Could you check a few things on this model? Use its own coordinates, in mm. Give positions to 0.01 mm unless a question says otherwise; leave off trailing zeros. Order: outer loops, then holes, each group sorted by start corner. A loop starts at its lowest first (then second) coordinate and runs counter-clockwise, first axis right, second up.
from build123d import *

# Parameters (mm, degrees)
EXTRUDE_1_DEPTH = 1.2


with BuildPart() as part:
    # 스케치1 → 보스-돌출1 (new body)
    with BuildSketch(Plane(origin=(0, 0, 0), x_dir=(1, 0, 0), z_dir=(0, 1, 0))):
        with BuildLine():
            Line((96.5, 48.995454452), (96.5, 85))
            ThreePointArc((96.5, 85), (93.863961031, 91.363961031), (87.5, 94))
            Line((87.5, 94), (-96.5, 94))
            Line((-96.5, 94), (-96.5, -95))
            Line((-96.5, -95), (-7.113574645, -95))
            ThreePointArc((-7.113574645, -95), (8.212657599, 3.247727485), (96.5, 48.995454452))
        make_face()
        with BuildLine():
            ThreePointArc((-86, -83), (-88, -81), (-86, -79))
            Line((-86, -79), (-84, -79))
            Line((-84, -79), (-82, -79))
            ThreePointArc((-82, -79), (-80.585786438, -79.585786438), (-80, -81))
            ThreePointArc((-80, -81), (-80.585786438, -82.414213562), (-82, -83))
            Line((-82, -83), (-84, -83))
            Line((-84, -83), (-86, -83))
        make_face(mode=Mode.SUBTRACT)
        with BuildLine():
            ThreePointArc((-86, -61), (-88, -59), (-86, -57))
            Line((-86, -57), (-84, -57))
            Line((-84, -57), (-82, -57))
            ThreePointArc((-82, -57), (-80.585786438, -57.585786438), (-80, -59))
            ThreePointArc((-80, -59), (-80.585786438, -60.414213562), (-82, -61))
            Line((-82, -61), (-84, -61))
            Line((-84, -61), (-86, -61))
        make_face(mode=Mode.SUBTRACT)
        with BuildLine():
            ThreePointArc((-86, 57), (-88, 59), (-86, 61))
            Line((-86, 61), (-84, 61))
            Line((-84, 61), (-82, 61))
            ThreePointArc((-82, 61), (-80.585786438, 60.414213562), (-80, 59))
            ThreePointArc((-80, 59), (-80.585786438, 57.585786438), (-82, 57))
            Line((-82, 57), (-84, 57))
            Line((-84, 57), (-86, 57))
        make_face(mode=Mode.SUBTRACT)
        with BuildLine():
            ThreePointArc((-86, 79), (-88, 81), (-86, 83))
            Line((-86, 83), (-84, 83))
            Line((-84, 83), (-82, 83))
            ThreePointArc((-82, 83), (-80.585786438, 82.414213562), (-80, 81))
            ThreePointArc((-80, 81), (-80.585786438, 79.585786438), (-82, 79))
            Line((-82, 79), (-84, 79))
            Line((-84, 79), (-86, 79))
        make_face(mode=Mode.SUBTRACT)
    extrude(amount=EXTRUDE_1_DEPTH)


solid = part.part
Item 1: Imagine slicing it at A-A on y = 0.9. List the corners of the cut face in (x, z) for me.
Findings:
outline: (-96.5, -94) - (87.5, -94) arc R9 ccw to (96.5, -85) - (96.5, -49) arc R110 cw to (-7.11, 95) - (-96.5, 95) - close; hole (-86, -83) - (-82, -83) arc R2 ccw to (-82, -79) - (-86, -79) arc R2 ccw to start; hole (-86, -61) - (-82, -61) arc R2 ccw to (-82, -57) - (-86, -57) arc R2 ccw to start; hole (-86, 57) - (-82, 57) arc R2 ccw to (-82, 61) - (-86, 61) arc R2 ccw to start; hole (-86, 79) - (-82, 79) arc R2 ccw to (-82, 83) - (-86, 83) arc R2 ccw to start
Item 2: Imagine slicing it at B-B on z = -10. List the corners of the cut face in (x, y) for me.
Findings:
outline: (-96.5, 0) - (13.48, 0) - (13.48, 1.2) - (-96.5, 1.2) - close
Item 3: Imagine slicing it at C-C on x = 61. List the corners of the cut face in (y, z) for me, then the cut area to 3 significant figures.
Findings:
outline: (0, -94) - (1.2, -94) - (1.2, -42.77) - (0, -42.77) - close
area: 61.5 mm2
Item 4: Please list where these lines run through material, in increasing order: line 1 along Z through (x, y) = (-86, 0.5); line 2 along X through (y, z) = (1.1, 59.5); line 3 along X through (y, z) = (1.15, 50).
Findings:
line 1: z = -94 to -83, -79 to -61, -57 to 57, 61 to 79, 83 to 95
line 2: x = -96.5 to -87.94, -80.06 to -12.49
line 3: x = -96.5 to -11.95
